Model file for the job. Use its own axes, mm. Face numbers are marked on the shaded views. A direction names the side the tool comes from. Coordinates: 2 decimals unless noted, no trailing zeros. Write each loop counter-clockwise with the first axis right and the second up, starting at its lowest first coordinate (ties: lowest second). Pieces come first, ordered by that corner, then holes.
Q1. Band-saw the part on A-A, the plane z = 90.5. Write the cut outline in (x, y).
Q2. Which spindle directions (+Z, -Z, +X, -X, +Y, -Y) get a long thin tool onto all of the face, cutting with end or side? Do the marked faces 1, 2 and 3. Say none if no direction does.
Q3. Drill centre lines: probe 1 along X at (y, z) = (2.1, 7.5); probe 2 along Y at (x, z) = (1.5, 47); probe 3 along Z at (x, y) = (0.5, 26). Where is each one in solid material? Low to high.
Q4. Pin check, flat tips, straight feed: P1, Ø2, axis at x = 3.25, z = 7.5, coming from the +Y side; P2, Ø5, axis at y = 6.5, z = 87.5, coming from the -X side; P3, Ø1.5, axis at x = -1.5, y = 0, coming from the -Z side; P4, Ø1.5, axis at x = 3, y = -6.5, coming from the -Z side. Stop position of each tip, or through.
Q5. Band-saw the part on B-B, the plane y = 3. Write the cut outline in (x, z).
Q6. Band-saw the part on C-C, the plane y = -11. Write the cut outline in (x, z).
Q7. Band-saw the part on D-D, the plane z = 50. Write the cut outline in (x, y).
from build123d import *
from build123d.topology import SkipClean

# Parameters (mm, degrees)
BOSS_EXTRUDE1_DEPTH      = 5
BOSS_EXTRUDE2_DEPTH      = 25
BOSS_EXTRUDE2_DEPTH_BACK = 50
FILLET1_R                = 20
SKETCH3_R                = 1.8
CUT_EXTRUDE1_DEPTH       = 19
SKETCH4_R                = 1.8
CUT_EXTRUDE2_DEPTH       = 10


with BuildPart() as part:
    # Sketch1 → Boss-Extrude1 (new body)
    with SkipClean():  # the faces are left unmerged after this step: merging them gives an invalid solid
        with BuildSketch(Plane(origin=(0, 0, 0), x_dir=(1, 0, 0), z_dir=(0, 1, 0))):
            with BuildLine():
                ThreePointArc((0, -0.740747083), (-3.176101933, -3.632802831), (-4.24425851, -7.793409934))
                Line((-4.24425851, -7.793409934), (0, -14.259252917))
                Line((0, -14.259252917), (0, -0.740747083))
            make_face()
            with BuildLine():
                Line((6, -0.522357132), (6, -14.477642868))
                Line((6, -14.477642868), (10.742827875, -7.827918338))
                ThreePointArc((10.742827875, -7.827918338), (10.748206754, -7.663998381), (10.75, -7.5))
                ThreePointArc((10.75, -7.5), (9.449798384, -3.279514246), (6, -0.522357132))
            make_face()
            with BuildLine():
                Line((0, -0.740747083), (0, -14.259252917))
                ThreePointArc((0, -14.259252917), (2.977193214, -14.995036788), (6, -14.477642868))
                Line((6, -14.477642868), (6, -0.522357132))
                ThreePointArc((6, -0.522357132), (4.649585383, -0.131746424), (3.25, 0))
                ThreePointArc((3.25, 0), (1.583326199, -0.187531303), (0, -0.740747083))
            make_face()
            with BuildLine():
                ThreePointArc((0, -14.259252917), (-3.019892671, -11.615634325), (-4.24425851, -7.793409934))
                Line((-4.24425851, -7.793409934), (0, -116.2))
                Line((0, -116.2), (0, -14.259252917))
            make_face()
            with BuildLine():
                Line((6, -14.477642868), (6, -116.2))
                Line((6, -116.2), (10.742827875, -7.827918338))
                ThreePointArc((10.742827875, -7.827918338), (9.356028972, -11.855044225), (6, -14.477642868))
            make_face()
            with BuildLine():
                Line((0, -14.259252917), (0, -116.2))
                Line((0, -116.2), (6, -116.2))
                Line((6, -116.2), (6, -14.477642868))
                ThreePointArc((6, -14.477642868), (2.977193214, -14.995036788), (0, -14.259252917))
            make_face()
            with BuildLine():
                Line((10.742827875, -7.827918338), (6, -14.477642868))
                ThreePointArc((6, -14.477642868), (9.356028972, -11.855044225), (10.742827875, -7.827918338))
            make_face()
            with BuildLine():
                Line((0, -14.259252917), (-4.24425851, -7.793409934))
                ThreePointArc((-4.24425851, -7.793409934), (-3.019892671, -11.615634325), (0, -14.259252917))
            make_face()
        extrude(amount=BOSS_EXTRUDE1_DEPTH)

    # Sketch2 → Boss-Extrude2 (add, two sides: drawn at the far end of the back side and taken through both)
    with BuildSketch(Plane(origin=(0, 5, 0), x_dir=(1, 0, 0), z_dir=(0, 1, 0)).offset(-BOSS_EXTRUDE2_DEPTH_BACK)):
        Polygon((-1.749928594, -71.503431366), (7.937559289, -71.927397454), (6, -116.2), (0, -116.2), align=None)
    extrude(amount=BOSS_EXTRUDE2_DEPTH + BOSS_EXTRUDE2_DEPTH_BACK)

    # Fillet1
    fillet1_edges = [part.edges().sort_by_distance(p)[0] for p in [
        (3.093815347, 5, 71.71541441),
        (3.093815347, 0, 71.71541441),
    ]]
    fillet(fillet1_edges, radius=FILLET1_R)

    # Sketch3 → Cut-Extrude1 (cut)
    with BuildSketch(Plane(origin=(0, 5, 0), x_dir=(1, 0, 0), z_dir=(0, 1, 0))):
        with Locations(Location((3.25, -7.5, 0), (0, 0, 270))):
            Circle(SKETCH3_R)
        with Locations(Location((4.169351127, -30.982009997, 0), (0, 0, 270))):
            Circle(SKETCH3_R)
    extrude(amount=-CUT_EXTRUDE1_DEPTH, mode=Mode.SUBTRACT)

    # Sketch4 → Cut-Extrude2 (cut)
    with BuildSketch(Plane(origin=(-4.542417883, 0, 0.177841548), x_dir=(0.03912132455492767, 0, 0.9992344679628841), z_dir=(-0.9992344679628841, 0, 0.03912132455492767))):
        with Locations((108.611045177, -40)):
            Circle(SKETCH4_R)
        with Locations((108.611045177, 25)):
            Circle(SKETCH4_R)
    extrude(amount=-CUT_EXTRUDE2_DEPTH, mode=Mode.SUBTRACT)


solid = part.part
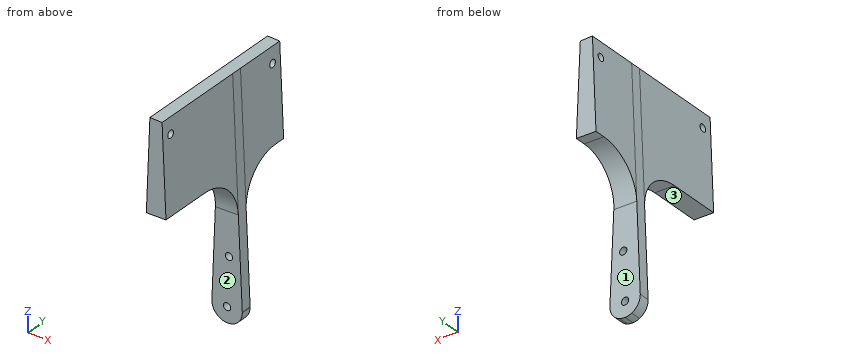
Answer sheet:
1. outline: (-1.01, -45) - (7.12, -45) - (7.12, 30) - (-1.01, 30) - close
2. face 1: -Z, +X, -X, +Y
2. face 2: -Z, +X, -X, -Y
2. face 3: -Z, +X, -Y
3. probe 1: x = -4.25 to 1.45, 5.05 to 10.75
3. probe 2: y = 0 to 5
3. probe 3: z = 71.6 to 107.18, 110.17 to 116.2
4. P1: passes through
4. P2: stops at x = -1.22
4. P3: stops at z = 1.16
4. P4: stops at z = 65.74
5. outline: (-4.24, 7.79) arc R7.5 ccw (long way) to (10.75, 7.5) arc R7.5 ccw to (10.74, 7.83) - (6, 116.2) - (0, 116.2) - close; hole circle Ø3.6 at (3.25, 7.5); hole circle Ø3.6 at (4.17, 30.98)
6. outline: (-1.83, 69.36) - (8.03, 69.79) - (6, 116.2) - (0, 116.2) - close
7. outline: (-2.59, 0) - (8.9, 0) - (8.9, 5) - (-2.59, 5) - close
